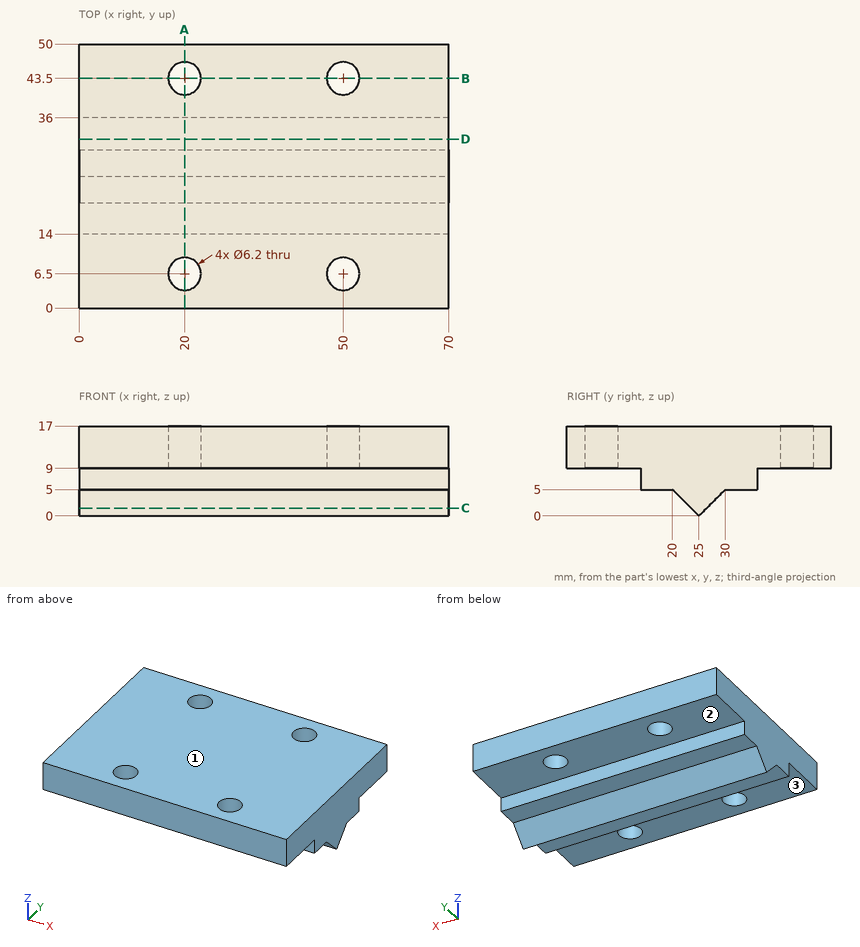
Could you check a few things on this drawing? It's one solid part, dimensions in mm from its lowest x, y, z. A direction names the side the tool comes from. Give positions to 0.01 mm unless a question says otherwise; leave off trailing zeros. Order: outer loops, then holes, each group sorted by start corner. A loop starts at its lowest first (then second) coordinate and runs counter-clockwise, first axis right, second up. Notation, with made-up numbers: (-35, 88.5) - (-9, 88.5) arc R8 ccw to (-9, 98.5) - close; hole circle Ø2 at (3.5, 78.5). An arc over 180 degrees is marked (long way). Return JSON: item names as keys, results as strings. Group by question number.
Q1. Suppose I cut it at A-A, the plane x = 20. Please give me the cut outline in (y, z), and give its area (3 significant figures).
Q2. Will these pins go through, and if not, where does the flat tip stop? pin 1 Ø3 at (x, z) = (37, 6.5) entering from -Y; pin 2 Ø1.8 at (x, y) = (27, 33) entering from -Z; pin 3 Ø3 at (x, y) = (47, 9) entering from -Z.
Q3. Suppose I cut it at C-C, the plane z = 1.5. Please give me the cut outline in (x, y).
Q4. Please list where these lines run through material, in increasing order: line 1 along Y through (x, z) = (20, 15.25); line 2 along Y through (x, z) = (21.5, 14.25); line 3 along Z through (x, y) = (23, 31.5). Write a range as [from, to].
Q5. Which directions (+Z, -Z, +X, -X, +Y, -Y) give clear straight access to the entire face, cutting with the end or side of a thin tool? Please do the marked faces 1, 2 and 3.
Q6. Suppose I cut it at B-B, the plane y = 43.5. Please give me the cut outline in (x, z).
Q7. Suppose I cut it at D-D, the plane y = 32. Please give me the cut outline in (x, z), and give its area (3 significant figures).
Resolved:
{
 "1": {"outline": "(0, 9) - (3.4, 9) - (3.4, 17) - (0, 17) - close; (9.6, 9) - (14, 9) - (14, 5) - (20, 5) - (25, 0) - (30, 5) - (36, 5) - (36, 9) - (40.4, 9) - (40.4, 17) - (9.6, 17) - close; (46.6, 9) - (50, 9) - (50, 17) - (46.6, 17) - close", "area": "414 mm2"},
 "2": {"pin 1": "stops at y = 14", "pin 2": "stops at z = 5", "pin 3": "stops at z = 9"},
 "3": {"outline": "(0, 23.5) - (70, 23.5) - (70, 26.5) - (0, 26.5) - close"},
 "4": {"line 1": "y = [0, 3.4], [9.6, 40.4], [46.6, 50]", "line 2": "y = [0, 3.79], [9.21, 40.79], [46.21, 50]", "line 3": "z = [5, 17]"},
 "5": {"face 1": "+Z, +X, -X, +Y, -Y", "face 2": "-Z, +X, -X, +Y", "face 3": "-Z, +X, -X, -Y"},
 "6": {"outline": "(0, 9) - (16.9, 9) - (16.9, 17) - (0, 17) - close; (23.1, 9) - (46.9, 9) - (46.9, 17) - (23.1, 17) - close; (53.1, 9) - (70, 9) - (70, 17) - (53.1, 17) - close"},
 "7": {"outline": "(0, 5) - (70, 5) - (70, 17) - (0, 17) - close", "area": "840 mm2"}
}
